from build123d import *

# Parameters (mm, degrees)
ESQUISSE15_R        = 1.5
BOSS_EXTRU_15_DEPTH = 3


with BuildPart() as part:
    # Esquisse15 → Boss.-Extru.15 (new body)
    with BuildSketch(Plane.XY):
        with BuildLine():
            Line((209.424329445, 31.309985915), (211.424329445, 31.309985915))
            Line((211.424329445, 31.309985915), (211.424329445, 35.309985915))
            Line((211.424329445, 35.309985915), (209.924329445, 35.309985915))
            Line((209.924329445, 35.309985915), (209.924329445, 37.809985915))
            Line((209.924329445, 37.809985915), (211.424329445, 37.809985915))
            Line((211.424329445, 37.809985915), (211.424329445, 41.309985915))
            Line((211.424329445, 41.309985915), (214.424329445, 41.309985915))
            Line((214.424329445, 41.309985915), (214.424329445, 37.809985915))
            Line((214.424329445, 37.809985915), (215.924329445, 37.809985915))
            Line((215.924329445, 37.809985915), (215.924329445, 35.309985915))
            Line((215.924329445, 35.309985915), (214.424329445, 35.309985915))
            Line((214.424329445, 35.309985915), (214.424329445, 31.309985915))
            Line((214.424329445, 31.309985915), (217.924329445, 31.309985915))
            Line((217.924329445, 31.309985915), (217.924329445, 32.809985915))
            Line((217.924329445, 32.809985915), (220.924329445, 32.809985915))
            Line((220.924329445, 32.809985915), (220.924329445, 42.809985915))
            Line((220.924329445, 42.809985915), (217.924329445, 42.809985915))
            Line((217.924329445, 42.809985915), (217.924329445, 47.029043611))
            Line((217.924329445, 47.029043611), (214.745710446, 59.763094048))
            ThreePointArc((214.745710446, 59.763094048), (209.355265644, 64.294490405), (203.371200864, 60.582157334))
            ThreePointArc((203.371200864, 60.582157334), (200.818725519, 56.947971615), (196.944306758, 54.777415122))
            Line((196.944306758, 54.777415122), (169.924329445, 46.809985915))
            Line((169.924329445, 46.809985915), (169.924329445, 42.809985915))
            Line((169.924329445, 42.809985915), (166.924329445, 42.809985915))
            Line((166.924329445, 42.809985915), (166.924329445, 32.809985915))
            Line((166.924329445, 32.809985915), (169.924329445, 32.809985915))
            Line((169.924329445, 32.809985915), (169.924329445, 31.309985915))
            Line((169.924329445, 31.309985915), (173.424329445, 31.309985915))
            Line((173.424329445, 31.309985915), (173.424329445, 35.309985915))
            Line((173.424329445, 35.309985915), (171.924329445, 35.309985915))
            Line((171.924329445, 35.309985915), (171.924329445, 37.809985915))
            Line((171.924329445, 37.809985915), (173.424329445, 37.809985915))
            Line((173.424329445, 37.809985915), (173.424329445, 41.309985915))
            Line((173.424329445, 41.309985915), (176.424329445, 41.309985915))
            Line((176.424329445, 41.309985915), (176.424329445, 37.809985915))
            Line((176.424329445, 37.809985915), (177.924329445, 37.809985915))
            Line((177.924329445, 37.809985915), (177.924329445, 35.309985915))
            Line((177.924329445, 35.309985915), (176.424329445, 35.309985915))
            Line((176.424329445, 35.309985915), (176.424329445, 31.309985915))
            Line((176.424329445, 31.309985915), (178.424329445, 31.309985915))
            Line((178.424329445, 31.309985915), (178.424329445, 32.809985915))
            Line((178.424329445, 32.809985915), (181.424329445, 32.809985915))
            Line((181.424329445, 32.809985915), (181.424329445, 33.809985915))
            Line((181.424329445, 33.809985915), (186.424329445, 33.809985915))
            Line((186.424329445, 33.809985915), (186.424329445, 36.309985915))
            Line((186.424329445, 36.309985915), (201.424329445, 36.309985915))
            Line((201.424329445, 36.309985915), (201.424329445, 33.809985915))
            Line((201.424329445, 33.809985915), (206.424329445, 33.809985915))
            Line((206.424329445, 33.809985915), (206.424329445, 32.809985915))
            Line((206.424329445, 32.809985915), (209.424329445, 32.809985915))
            Line((209.424329445, 32.809985915), (209.424329445, 31.309985915))
        make_face()
        with Locations((208.924329445, 58.309985915)):
            Circle(ESQUISSE15_R, mode=Mode.SUBTRACT)
    extrude(amount=BOSS_EXTRU_15_DEPTH)


solid = part.part
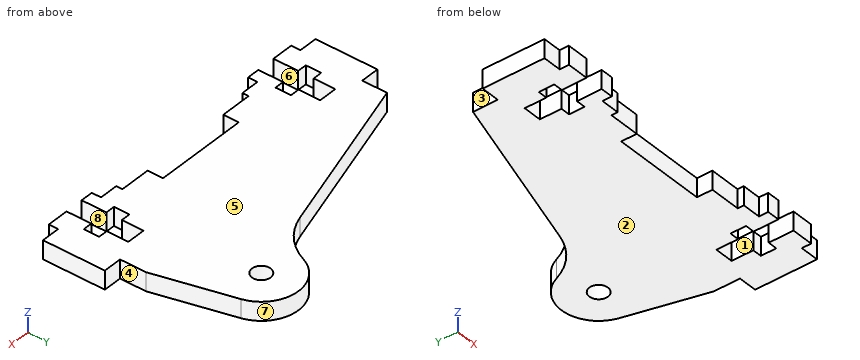
Model file for the job. Use its own axes, mm. Face numbers are marked on the shaded views. A direction names the side the tool comes from. Give positions to 0.01 mm unless a question says otherwise; leave off trailing zeros. Loops run counter-clockwise (first coordinate to the right, second up) from the corner with the lowest first, then second, coordinate; pieces in that order, holes last. Notation, with made-up numbers: (17.25, -22) -> (46.25, -22) arc R37 ccw to (46.25, 17) -> close; hole circle Ø2 at (23.25, 80.25). An arc over 180 degrees is marked (long way). Use a Markdown table: item, result. Add a question column.
(1) Mould opens along X. For the marked faces 5, 6, 7 and 8 say: +X half, -X half, draft (parallel to the pull), parting line (faces both ways), or undercut.
(2) Drop flat-ended pins along their axis: pin 1 Ø1.2 at (x, z) = (173, 1.5) entering from +Y; pin 2 Ø0.9 at (x, z) = (212.5, 1.5) entering from -Y; pin 3 Ø1.5 at (x, z) = (207.5, 2) entering from -Y. Give the stop position or say it passes through.
(3) Slice it at B-B on x = 217. List the corners of the cut face in (y, z).
(4) Tool access for the marked faces 1, 2, 3 and 4: list every direction of +Z, -Z, +X, -X, +Y, -Y with a clear straight run to the whole face (end or side of a thin tool).
(5) Wall check: line 1 along X through (y, z) = (33, 1.6); line 2 along X through (y, z) = (38, 1.8); line 3 along Y through (x, z) = (208.5, 2.6). Give the ranges that are in metal, low to high.
(6) Slice it at A-A on y = 45. List the corners of the cut face in (x, z), and give its area (3 significant figures).
Filled sheet:
| question | item | result |
|---|---|---|
| 1 | face 5 | draft |
| 1 | face 6 | undercut |
| 1 | face 7 | parting line |
| 1 | face 8 | undercut |
| 2 | pin 1 | y = 47.89 |
| 2 | pin 2 | y = 41.31 |
| 2 | pin 3 | y = 32.81 |
| 3 | outline | (31.31, 0) -> (50.73, 0) -> (50.73, 3) -> (31.31, 3) -> close |
| 4 | face 1 | +Z, -Z, -Y |
| 4 | face 2 | -Z, +X, -X, +Y, -Y |
| 4 | face 3 | +Z, -Z, -X, +Y |
| 4 | face 4 | +Z, -Z, +X, +Y |
| 5 | line 1 | 166.92 to 173.42, 176.42 to 181.42, 206.42 to 211.42, 214.42 to 220.92 |
| 5 | line 2 | 166.92 to 173.42, 176.42 to 211.42, 214.42 to 220.92 |
| 5 | line 3 | 32.81 to 56.87, 59.75 to 64.29 |
| 6 | outline | (169.92, 0) -> (217.92, 0) -> (217.92, 3) -> (169.92, 3) -> close |
| 6 | area | 144 mm2 |
